Geometry: final body of the model. Coordinates: model frame, mm. A direction names the side the tool comes from. Round coordinates to 2 decimals unless told otherwise and drop trailing zeros. Loops run counter-clockwise (first coordinate to the right, second up) from the corner with the lowest first, then second, coordinate; pieces in that order, holes last. Notation, with made-up numbers: (85.25, 35) - (112.25, 35) arc R27 cw to (112.25, 55) - close; hole circle Ø8 at (-21, 55.25). An arc over 180 degrees is marked (long way). Answer as CSV lines item,"result".
from build123d import *

# Parameters (mm, degrees)
F0_R     = 12.7
F0_R_2   = 10.16
F0_R_3   = 6.731
F1_DEPTH = 6.3754
F2_DEPTH = 2.54
F3_DEPTH = 1.27
F4_SIZE  = 1.6002


with BuildPart() as f1:
    # F0 (on Top) → F1 (new body)
    with BuildSketch(Plane.XY):
        Circle(F0_R)
        Circle(F0_R_2, mode=Mode.SUBTRACT)
        Circle(F0_R_2)
        Circle(F0_R_3, mode=Mode.SUBTRACT)
        Circle(F0_R_3)
    extrude(amount=F1_DEPTH)

    # F0 (on Top) → F2 (cut)
    with BuildSketch(Plane.XY):
        Circle(F0_R)
        Circle(F0_R_2, mode=Mode.SUBTRACT)
    extrude(amount=F2_DEPTH, mode=Mode.SUBTRACT)

    # F0 (on Top) → F3 (cut)
    with BuildSketch(Plane.XY):
        Circle(F0_R_3)
    extrude(amount=F3_DEPTH, mode=Mode.SUBTRACT)

    # F4
    f4_edges = [f1.edges().sort_by_distance(p)[0] for p in [
        (-12.7, 0, 6.3754),
    ]]
    chamfer(f4_edges, length=F4_SIZE)


solid = f1.part
(1) Material intervals for line 1 along Y through (x, z) = (0, 0.75); line 2 along Z through (x, y) = (4.25, 2.25); line 3 along Y through (x, z) = (-5.25, 5.75), sorted ascending.
Findings below:
line 1,"-10.16 to -6.73, 6.73 to 10.16"
line 2,"1.27 to 6.38"
line 3,"-10.48 to 10.48"
(2) Draft query along X for faces 3 (the face through (-5.34, -4.1, 0.63)), 4 (the face through (0, 0, 6.375)), 5 (the face through (-1.323, 10.074, 1.252)). Return one class per face: pulls with the +X half, pulls with the -X half, needs draft (parallel to the pull), parting line crosses it, or undercut.
Findings below:
face 3,"undercut"
face 4,"needs draft"
face 5,"parting line crosses it"
(3) Pin query (flat end, axial travel): P1, Ø1.5, axis at y = 3.5, z = 2.5, coming from the +X side; P2, Ø1.5, axis at y = -1, z = 2, coming from the +X side; P3, Ø3, axis at x = 3.5, z = 3.5, coming from the +Y side; P4, Ø15, axis at x = -2, y = 2, coming from the -Z side. Return the tip coordinate at first contact, or that it passes through.
Findings below:
P1,"x = 12.4"
P2,"x = 12.69"
P3,"y = 12.54"
P4,"z = 0"
(4) Access query for faces 1 (the face through (-2.75, -12.4, 3.64)), 2 (the face through (0, 0, 1.27)). Directions: +Z, -Z, +X, -X, +Y, -Y. A direction counts if a zero-diameter tool reaches every point of the face in a straight line with its end or side. Return the directions, or none.
Findings below:
face 1,"+Z, -Z"
face 2,"-Z"
(5) Section D-D (z = 0.5). Output: boundary loops of the cut face in (x, y), and give its area (3 significant figures).
Findings below:
outline,"circle Ø20.32 at (0, 0); hole circle Ø13.46 at (0, 0)"
area,"182 mm2"
(6) Section C-C (z = 3.5). Output: boundary loops of the cut face in (x, y).
Findings below:
outline,"circle Ø25.4 at (0, 0)"
(7) Section A-A (x = 0). Output: boundary loops of the cut face in (y, z).
Findings below:
outline,"(-12.7, 2.54) - (-10.16, 2.54) - (-10.16, 0) - (-6.73, 0) - (-6.73, 1.27) - (6.73, 1.27) - (6.73, 0) - (10.16, 0) - (10.16, 2.54) - (12.7, 2.54) - (12.7, 4.78) - (11.1, 6.38) - (-11.1, 6.38) - (-12.7, 4.78) - close"
